Input: part model. Units: mm. Frame: model coordinates. Round coordinates to 2 decimals unless told otherwise and drop trailing zeros. Loops run counter-clockwise (first coordinate to the right, second up) from the corner with the lowest first, then second, coordinate; pieces in that order, holes last. Notation, with made-up numbers: (23.5, -13) - (37.5, -13) arc R23 ccw to (37.5, 11) - close; hole circle Ø5 at (-8.75, 88.25). An arc over 180 degrees is marked (long way). Write each question's results on one line, items separated by ' | '.
Autodesk Inventor part; units mm, degrees
ref_plane "YZ Plane" through (0, 0, 0) normal (1, 0, 0) x (0, 1, 0)
ref_plane "XZ Plane" through (0, 0, 0) normal (0, 1, 0) x (-1, 0, 0)
ref_plane "XY Plane" through (0, 0, 0) normal (0, 0, 1) x (1, 0, 0)
sketch "Sketch1" plane through (0, 0, 0) normal (0, 0, 1) x (1, 0, 0)
  line L0 (0, 0) -> (742.95, 0)
  line L1 (742.95, 0) -> (742.95, 38.1)
  line L2 (742.95, 38.1) -> (0, 38.1)
  line L3 (0, 38.1) -> (0, 0)
  dimension "d0" = 742.95
  dimension "d1" = 38.1
extrude "Board" add sketch "Sketch1" along normal blind 19.05
sketch "Sketch2" plane through (0, 0, 19.05) normal (0, 0, 1) x (1, 0, 0)
  line L0 (742.95, 38.1) -> (0, 38.1)
  line L1 (0, 0) -> (742.95, 0)
  line L2 (352.425, 38.1) -> (390.525, 38.1)
  line L3 (390.525, 38.1) -> (390.525, 0)
  line L4 (390.525, 0) -> (352.425, 0)
  line L5 (352.425, 0) -> (352.425, 38.1)
  line L6 (0, 38.1) -> (0, 0)
  dimension "d4" = 38.1
  dimension "d5" = 352.425
extrude "Extrusion2" cut sketch "Sketch2" against normal blind 9.525 contours L3 L1 L5 L0
equation "\"d5\" = -0.5 * d4 + 0.5 * d0"
properties part number "Cabinet Support Frame Horizontal Bar Low"
1. Section query A-A, the plane z = 15.25. Output: boundary loops of the cut face in (x, y) (3 decimals).
Answer:
outline: (0, 0) - (352.425, 0) - (352.425, 38.1) - (0, 38.1) - close; (390.525, 0) - (742.95, 0) - (742.95, 38.1) - (390.525, 38.1) - close
2. Mould query, pull axis X, two halves, no side actions, for faces 1 (the flat face through (371, 19, 9.525)), 2 (the flat face through (0, 19, 9)), 3 (the flat face through (174, 19, 19.05)). Classes: pulls with the +X half, pulls with the -X half, needs draft (parallel to the pull), parting line crosses it, or undercut.
Answer:
face 1: undercut | face 2: pulls with the -X half | face 3: needs draft
3. Section query B-B, the plane y = 24. Output: boundary loops of the cut face in (x, z) (3 decimals), plus the area to 3 significant figures.
Answer:
outline: (0, 0) - (742.95, 0) - (742.95, 19.05) - (390.525, 19.05) - (390.525, 9.525) - (352.425, 9.525) - (352.425, 19.05) - (0, 19.05) - close | area: 13,800 mm^2
4. Line query: line 1 (X direction, y = 20.5, z = 13.5) (3 decimals); line 2 (Z direction, x = 390, y = 17.5) (3 decimals). Output: solid intervals per line, ascending. Write a range as [from, to].
Answer:
line 1: [0, 352.425], [390.525, 742.95] | line 2: [0, 9.525]
